Autodesk Inventor part; units mm, degrees
ref_plane "YZ Plane" through (0, 0, 0) normal (1, 0, 0) x (0, 1, 0)
ref_plane "XZ Plane" through (0, 0, 0) normal (0, 1, 0) x (-1, 0, 0)
ref_plane "XY Plane" through (0, 0, 0) normal (0, 0, 1) x (1, 0, 0)
sketch "Sketch1" plane through (0, 0, 0) normal (0, 1, 0) x (-1, 0, 0)
  line L0 (0, 0) -> (230, 0)
  line L1 (230, 0) -> (230, -230)
  line L2 (230, -230) -> (0, -230)
  line L3 (0, -230) -> (0, 0)
  dimension "d0" = 230
  dimension "d1" = 230
extrude "Extrusion1" add sketch "Sketch1" along normal blind 5
sketch "Sketch2" plane through (0, 5, 0) normal (0, 1, 0) x (1, 0, 0)
  line L0 (-215, 215) -> (-15, 215)
  line L1 (-15, 215) -> (-15, 15)
  line L2 (-15, 15) -> (-215, 15)
  line L3 (-215, 15) -> (-215, 215)
  line L4 (-230, 230) -> (-230, 0)
  point P0 (0, 0)
  dimension "d4" = 200
  dimension "d5" = 200
  dimension "d6" = 15
  dimension "d7" = 15
extrude "Extrusion2" cut sketch "Sketch2" against normal blind 2
chamfer "Chamfer1" distance 2 angle 45 4 edges at (-230, 2.5, 0) (-230, 2.5, -230) (0, 2.5, -230) (0, 2.5, 0)
properties part number "MouldBase20"
Read the model definition and answer for the solid it produces. Units are mm, in the model's axes. Coordinates: 2 decimals unless noted, no trailing zeros. Write each loop counter-clockwise with the first axis right and the second up, starting at its lowest first coordinate (ties: lowest second). Pieces come first, ordered by that corner, then holes. Notation, with made-up numbers: (79, -2) -> (98, -2) arc R27 ccw to (98, 22) -> close; hole circle Ø6 at (-9, -22.75). An arc over 180 degrees is marked (long way). Return JSON: item names as keys, results as strings.
(1) The part is cut by section A-A on x = -66. Give the vertices of the cut face in (y, z), then the cut area to 3 significant figures.
Answers below:
{"outline": "(0, -230) -> (5, -230) -> (5, -215) -> (3, -215) -> (3, -15) -> (5, -15) -> (5, 0) -> (0, 0) -> close", "area": "750 mm^2"}
(2) For a pull along Z with two mould halves and no side action, classify faces 1 (the flat face through (-11, 5, -113)), 2 (the flat face through (-117, 2, -230)), 3 (the flat face through (-116, 3, -116)), 4 (the flat face through (-113, 2, 0)) as pulls with the +Z half, pulls with the -Z half, needs draft (parallel to the pull), parting line crosses it, or undercut.
Answers below:
{"face 1": "needs draft", "face 2": "pulls with the -Z half", "face 3": "undercut", "face 4": "pulls with the +Z half"}
(3) Each of these flat-tipped pins is pushed along its axis until it touches: P1, Ø8, axis at x = -53.5, z = -71.5, coming from the +Y side; P2, Ø0.6, axis at y = 4.5, z = -103, coming from the +X side. Where does it stop, or does it pass through?
Answers below:
{"P1": "y = 3", "P2": "x = 0"}
(4) Consider line 1 along X through (y, z) = (3.3, -119); line 2 along Y through (x, z) = (-203.5, -93). Determine where each line is inside the solid, lowest interval first. Write a range as from..to.
Answers below:
{"line 1": "-230..-215, -15..0", "line 2": "0..3"}
(5) The part is cut by section B-B on y = 3.9. Give the vertices of the cut face in (x, z), then the cut area to 3 significant figures.
Answers below:
{"outline": "(-230, -228) -> (-228, -230) -> (-2, -230) -> (0, -228) -> (0, -2) -> (-2, 0) -> (-228, 0) -> (-230, -2) -> close; hole (-215, -215) -> (-15, -215) -> (-15, -15) -> (-215, -15) -> close", "area": "12,900 mm^2"}
(6) The part is cut by section C-C on z = -19. Give the vertices of the cut face in (x, y), then the cut area to 3 significant figures.
Answers below:
{"outline": "(-230, 0) -> (0, 0) -> (0, 5) -> (-15, 5) -> (-15, 3) -> (-215, 3) -> (-215, 5) -> (-230, 5) -> close", "area": "750 mm^2"}
